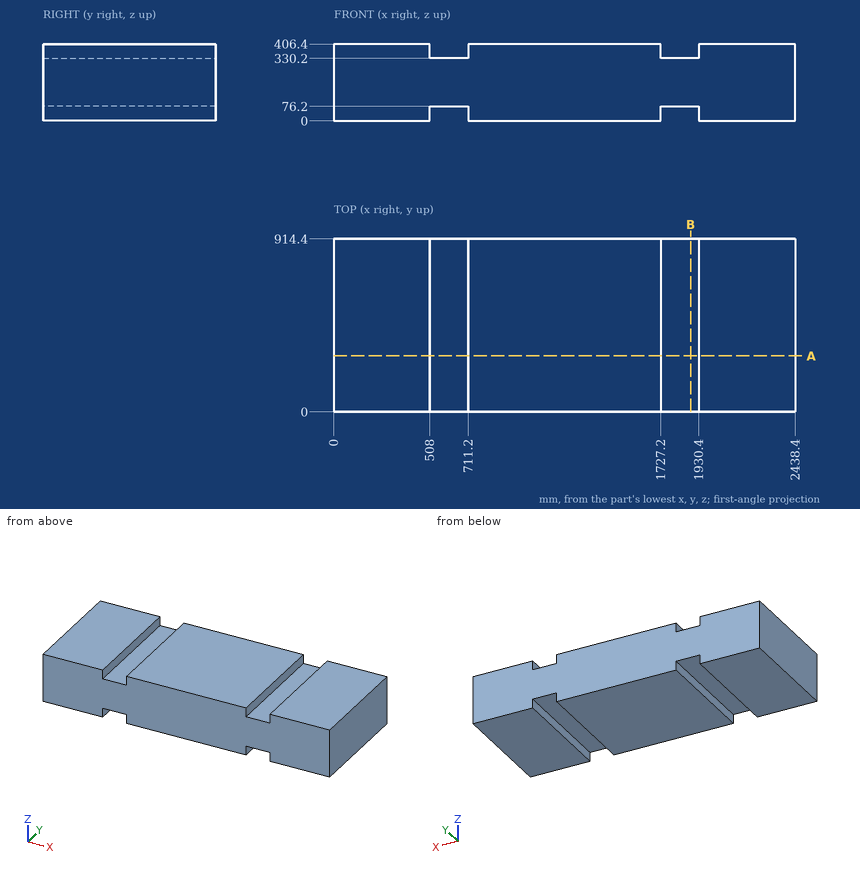
For this review, use the dimensioned drawing (mm, ordinates from the lowest corner) and the shaded views. Coordinates: 2 decimals unless noted, no trailing zeros. Order: outer loops, then holes, each group sorted by start corner. A loop starts at its lowest first (then second) coordinate and runs counter-clockwise, first axis right, second up. Notation, with made-up numbers: (-27, 13.5) -> (27, 13.5) arc R22 cw to (27, 28.5) -> close; hole circle Ø1 at (-10, 87.25). An arc over 180 degrees is marked (long way). One line per item, written item: value. Start each with the question number.
Q1. Take a section at B-B, the plane x = 1886.5. State the section outline as (y, z) points, then the cut area to 3 significant figures.
Q2. For probe 1 along X at (y, z) = (651.5, 356); probe 2 along Z at (x, y) = (1830.5, 649), list the stretches that pass through material, from the lowest coordinate up.
Q3. Take a section at A-A, the plane y = 295. State the section outline as (x, z) points.
Values follow:
1. outline: (0, 76.2) -> (914.4, 76.2) -> (914.4, 330.2) -> (0, 330.2) -> close
1. area: 232,000 mm2
2. probe 1: x = 0 to 508, 711.2 to 1727.2, 1930.4 to 2438.4
2. probe 2: z = 76.2 to 330.2
3. outline: (0, 0) -> (508, 0) -> (508, 76.2) -> (711.2, 76.2) -> (711.2, 0) -> (1727.2, 0) -> (1727.2, 76.2) -> (1930.4, 76.2) -> (1930.4, 0) -> (2438.4, 0) -> (2438.4, 406.4) -> (1930.4, 406.4) -> (1930.4, 330.2) -> (1727.2, 330.2) -> (1727.2, 406.4) -> (711.2, 406.4) -> (711.2, 330.2) -> (508, 330.2) -> (508, 406.4) -> (0, 406.4) -> close
